from build123d import *

# Parameters (mm, degrees)
CYLINDER1189_R               = 1.5
CYLINDER1189_DEPTH           = 100
CYLINDER1190_R               = 1.5
CYLINDER1190_DEPTH           = 100
CYLINDER1187_R               = 1.5
CYLINDER1187_DEPTH           = 100
CYLINDER1188_R               = 1.5
CYLINDER1188_DEPTH           = 100
BOX491_W                     = 2
BOX491_H                     = 6
BOX491_DEPTH                 = 6
BOX492_W                     = 2
BOX492_H                     = 6
BOX492_DEPTH                 = 6
BOX493_W                     = 2
BOX493_H                     = 6
BOX493_DEPTH                 = 6
BOX490_W                     = 2
BOX490_H                     = 6
BOX490_DEPTH                 = 6
BOX460_W                     = 8
BOX460_H                     = 6
BOX460_DEPTH                 = 2
BOX460_PLACEMENT_ANGLE       = 45
BOX461_W                     = 8
BOX461_H                     = 6
BOX461_DEPTH                 = 2
BOX462_W                     = 8
BOX462_H                     = 6
BOX462_DEPTH                 = 2
BOX462_PLACEMENT_ANGLE       = 135
BOX463_W                     = 8
BOX463_H                     = 6
BOX463_DEPTH                 = 2
BOX464_W                     = 8
BOX464_H                     = 6
BOX464_DEPTH                 = 2
BOX464_PLACEMENT_ANGLE       = 225
BOX465_W                     = 8
BOX465_H                     = 6
BOX465_DEPTH                 = 2
BOX466_W                     = 8
BOX466_H                     = 6
BOX466_DEPTH                 = 2
BOX466_PLACEMENT_ANGLE       = 45
BOX459_W                     = 8
BOX459_H                     = 6
BOX459_DEPTH                 = 2
CYLINDER1161_R               = 1.5
CYLINDER1161_DEPTH           = 50
CYLINDER1161_PLACEMENT_ANGLE = 45
CYLINDER1162_R               = 1.5
CYLINDER1162_DEPTH           = 50
CYLINDER1163_R               = 1.5
CYLINDER1163_DEPTH           = 50
CYLINDER1163_PLACEMENT_ANGLE = 135
CYLINDER1164_R               = 1.5
CYLINDER1164_DEPTH           = 50
CYLINDER1165_R               = 1.5
CYLINDER1165_DEPTH           = 50
CYLINDER1165_PLACEMENT_ANGLE = 225
CYLINDER1166_R               = 1.5
CYLINDER1166_DEPTH           = 50
CYLINDER1167_R               = 1.5
CYLINDER1167_DEPTH           = 50
CYLINDER1167_PLACEMENT_ANGLE = 45
CYLINDER1160_R               = 1.5
CYLINDER1160_DEPTH           = 50
TUBE109_R                    = 50
TUBE109_R_2                  = 40
TUBE109_DEPTH                = 11
TUBE107_R                    = 54
TUBE107_R_2                  = 47
TUBE107_DEPTH                = 25


with BuildPart() as obj1:
    # Cylinder1189 → Cylinder1189 (new body)
    with BuildSketch(Plane(origin=(24, -51, 27), x_dir=(0, 0, -1), z_dir=(1, 0, 0))):
        Circle(CYLINDER1189_R)
    extrude(amount=CYLINDER1189_DEPTH)


with BuildPart() as obj2:
    # Cylinder1190 → Cylinder1190 (new body)
    with BuildSketch(Plane(origin=(34, 36, 42), x_dir=(0, 0, -1), z_dir=(1, 0, 0))):
        Circle(CYLINDER1190_R)
    extrude(amount=CYLINDER1190_DEPTH)


with BuildPart() as obj3:
    # Cylinder1187 → Cylinder1187 (new body)
    with BuildSketch(Plane(origin=(34, -36, 42), x_dir=(0, 0, -1), z_dir=(1, 0, 0))):
        Circle(CYLINDER1187_R)
    extrude(amount=CYLINDER1187_DEPTH)


with BuildPart() as compound890:
    # Cylinder1188 → Cylinder1188 (new body)
    with BuildSketch(Plane(origin=(24, 51, 27), x_dir=(0, 0, -1), z_dir=(1, 0, 0))):
        Circle(CYLINDER1188_R)
    extrude(amount=CYLINDER1188_DEPTH)

    # Compound890: union obj1, obj2, obj3
    add(obj1.part)
    add(obj2.part)
    add(obj3.part)


with BuildPart() as krychle491:
    # Box491 → Box491 (new body)
    with BuildSketch(Plane(origin=(32, -54, 24), x_dir=(1, 0, 0), z_dir=(0, 0, 1))):
        with Locations((1, 3)):
            Rectangle(BOX491_W, BOX491_H)
    extrude(amount=BOX491_DEPTH)


with BuildPart() as krychle492:
    # Box492 → Box492 (new body)
    with BuildSketch(Plane(origin=(38, 33, 39), x_dir=(1, 0, 0), z_dir=(0, 0, 1))):
        with Locations((1, 3)):
            Rectangle(BOX492_W, BOX492_H)
    extrude(amount=BOX492_DEPTH)


with BuildPart() as krychle493:
    # Box493 → Box493 (new body)
    with BuildSketch(Plane(origin=(38, -39, 39), x_dir=(1, 0, 0), z_dir=(0, 0, 1))):
        with Locations((1, 3)):
            Rectangle(BOX493_W, BOX493_H)
    extrude(amount=BOX493_DEPTH)


with BuildPart() as compound888:
    # Box490 → Box490 (new body)
    with BuildSketch(Plane(origin=(32, 48, 24), x_dir=(1, 0, 0), z_dir=(0, 0, 1))):
        with Locations((1, 3)):
            Rectangle(BOX490_W, BOX490_H)
    extrude(amount=BOX490_DEPTH)

    # Compound888: union Krychle491, Krychle492, Krychle493
    add(krychle491.part)
    add(krychle492.part)
    add(krychle493.part)


with BuildPart() as krychle460:
    # Box460 → Box460 (new body)
    with BuildSketch(Plane.XY):
        with Locations((4, 3)):
            Rectangle(BOX460_W, BOX460_H)
    extrude(amount=BOX460_DEPTH)


with BuildPart() as krychle460_1:
    # Box460 placement: moved
    add(krychle460.part.moved(Location((35.355339, 31.112698, 34))).rotate(Axis((35.355339, 31.112698, 34), (0, 0, 1)), BOX460_PLACEMENT_ANGLE))


with BuildPart() as krychle461:
    # Box461 → Box461 (new body)
    with BuildSketch(Plane(origin=(3, 47, 34), x_dir=(0, 1, 0), z_dir=(0, 0, 1))):
        with Locations((4, 3)):
            Rectangle(BOX461_W, BOX461_H)
    extrude(amount=BOX461_DEPTH)


with BuildPart() as krychle462:
    # Box462 → Box462 (new body)
    with BuildSketch(Plane.XY):
        with Locations((4, 3)):
            Rectangle(BOX462_W, BOX462_H)
    extrude(amount=BOX462_DEPTH)


with BuildPart() as krychle462_1:
    # Box462 placement: moved
    add(krychle462.part.moved(Location((-31.112698, 35.355339, 34))).rotate(Axis((-31.112698, 35.355339, 34), (0, 0, 1)), BOX462_PLACEMENT_ANGLE))


with BuildPart() as krychle463:
    # Box463 → Box463 (new body)
    with BuildSketch(Plane(origin=(-47, 3, 34), x_dir=(-1, 0, 0), z_dir=(0, 0, 1))):
        with Locations((4, 3)):
            Rectangle(BOX463_W, BOX463_H)
    extrude(amount=BOX463_DEPTH)


with BuildPart() as krychle464:
    # Box464 → Box464 (new body)
    with BuildSketch(Plane.XY):
        with Locations((4, 3)):
            Rectangle(BOX464_W, BOX464_H)
    extrude(amount=BOX464_DEPTH)


with BuildPart() as krychle464_1:
    # Box464 placement: moved
    add(krychle464.part.moved(Location((-35.355339, -31.112698, 34))).rotate(Axis((-35.355339, -31.112698, 34), (0, 0, 1)), BOX464_PLACEMENT_ANGLE))


with BuildPart() as krychle465:
    # Box465 → Box465 (new body)
    with BuildSketch(Plane(origin=(-3, -47, 34), x_dir=(0, -1, 0), z_dir=(0, 0, 1))):
        with Locations((4, 3)):
            Rectangle(BOX465_W, BOX465_H)
    extrude(amount=BOX465_DEPTH)


with BuildPart() as krychle466:
    # Box466 → Box466 (new body)
    with BuildSketch(Plane.XY):
        with Locations((4, 3)):
            Rectangle(BOX466_W, BOX466_H)
    extrude(amount=BOX466_DEPTH)


with BuildPart() as krychle466_1:
    # Box466 placement: moved
    add(krychle466.part.moved(Location((31.112698, -35.355339, 34))).rotate(Axis((31.112698, -35.355339, 34), (0, 0, -1)), BOX466_PLACEMENT_ANGLE))


with BuildPart() as compound881:
    # Box459 → Box459 (new body)
    with BuildSketch(Plane(origin=(47, -3, 34), x_dir=(1, 0, 0), z_dir=(0, 0, 1))):
        with Locations((4, 3)):
            Rectangle(BOX459_W, BOX459_H)
    extrude(amount=BOX459_DEPTH)

    # Compound881: union Krychle460, Krychle461, Krychle462, Krychle463, Krychle464, Krychle465, Krychle466
    add(krychle460_1.part)
    add(krychle461.part)
    add(krychle462_1.part)
    add(krychle463.part)
    add(krychle464_1.part)
    add(krychle465.part)
    add(krychle466_1.part)


with BuildPart() as compound881_1:
    # Compound881 placement: moved
    add(compound881.part.moved(Location((0, 0, 1))))


with BuildPart() as obj4:
    # Cylinder1161 → Cylinder1161 (new body)
    with BuildSketch(Plane.XY):
        Circle(CYLINDER1161_R)
    extrude(amount=CYLINDER1161_DEPTH)


with BuildPart() as obj4_1:
    # Cylinder1161 placement: moved
    add(obj4.part.moved(Location((36.769553, 36.769553, 0))).rotate(Axis((36.769553, 36.769553, 0), (0, 0, 1)), CYLINDER1161_PLACEMENT_ANGLE))


with BuildPart() as obj5:
    # Cylinder1162 → Cylinder1162 (new body)
    with BuildSketch(Plane(origin=(0, 52, 0), x_dir=(0, 1, 0), z_dir=(0, 0, 1))):
        Circle(CYLINDER1162_R)
    extrude(amount=CYLINDER1162_DEPTH)


with BuildPart() as obj6:
    # Cylinder1163 → Cylinder1163 (new body)
    with BuildSketch(Plane.XY):
        Circle(CYLINDER1163_R)
    extrude(amount=CYLINDER1163_DEPTH)


with BuildPart() as obj6_1:
    # Cylinder1163 placement: moved
    add(obj6.part.moved(Location((-36.769553, 36.769553, 0))).rotate(Axis((-36.769553, 36.769553, 0), (0, 0, 1)), CYLINDER1163_PLACEMENT_ANGLE))


with BuildPart() as obj7:
    # Cylinder1164 → Cylinder1164 (new body)
    with BuildSketch(Plane(origin=(-52, 0, 0), x_dir=(-1, 0, 0), z_dir=(0, 0, 1))):
        Circle(CYLINDER1164_R)
    extrude(amount=CYLINDER1164_DEPTH)


with BuildPart() as obj8:
    # Cylinder1165 → Cylinder1165 (new body)
    with BuildSketch(Plane.XY):
        Circle(CYLINDER1165_R)
    extrude(amount=CYLINDER1165_DEPTH)


with BuildPart() as obj8_1:
    # Cylinder1165 placement: moved
    add(obj8.part.moved(Location((-36.769553, -36.769553, 0))).rotate(Axis((-36.769553, -36.769553, 0), (0, 0, 1)), CYLINDER1165_PLACEMENT_ANGLE))


with BuildPart() as obj9:
    # Cylinder1166 → Cylinder1166 (new body)
    with BuildSketch(Plane(origin=(0, -52, 0), x_dir=(0, -1, 0), z_dir=(0, 0, 1))):
        Circle(CYLINDER1166_R)
    extrude(amount=CYLINDER1166_DEPTH)


with BuildPart() as obj10:
    # Cylinder1167 → Cylinder1167 (new body)
    with BuildSketch(Plane.XY):
        Circle(CYLINDER1167_R)
    extrude(amount=CYLINDER1167_DEPTH)


with BuildPart() as obj10_1:
    # Cylinder1167 placement: moved
    add(obj10.part.moved(Location((36.769553, -36.769553, 0))).rotate(Axis((36.769553, -36.769553, 0), (0, 0, -1)), CYLINDER1167_PLACEMENT_ANGLE))


with BuildPart() as compound879:
    # Cylinder1160 → Cylinder1160 (new body)
    with BuildSketch(Plane(origin=(52, 0, 0), x_dir=(1, 0, 0), z_dir=(0, 0, 1))):
        Circle(CYLINDER1160_R)
    extrude(amount=CYLINDER1160_DEPTH)

    # Compound879: union obj4, obj5, obj6, obj7, obj8, obj9, obj10
    add(obj4_1.part)
    add(obj5.part)
    add(obj6_1.part)
    add(obj7.part)
    add(obj8_1.part)
    add(obj9.part)
    add(obj10_1.part)


with BuildPart() as compound879_1:
    # Compound879 placement: moved
    add(compound879.part.moved(Location((0, 0, -7))))


with BuildPart() as tube109:
    # Tube109 → Tube109 (new body)
    with BuildSketch(Plane.XY.offset(20)):
        Circle(TUBE109_R)
        Circle(TUBE109_R_2, mode=Mode.SUBTRACT)
    extrude(amount=TUBE109_DEPTH)


with BuildPart() as cut444:
    # Tube107 → Tube107 (new body)
    with BuildSketch(Plane.XY.offset(20)):
        Circle(TUBE107_R)
        Circle(TUBE107_R_2, mode=Mode.SUBTRACT)
    extrude(amount=TUBE107_DEPTH)

    # Cut429: cut Tube109
    add(tube109.part, mode=Mode.SUBTRACT)

    # Cut431: cut Compound879
    add(compound879_1.part, mode=Mode.SUBTRACT)

    # Cut432: cut Compound881
    add(compound881_1.part, mode=Mode.SUBTRACT)

    # Cut442: cut Compound888
    add(compound888.part, mode=Mode.SUBTRACT)

    # Cut444: cut Compound890
    add(compound890.part, mode=Mode.SUBTRACT)


solid = cut444.part
Source: CAD feature listing. Evaluate the final solid. Frame: model axes, mm. A direction names the side the tool comes from. Coordinates: 2 decimals unless noted, no trailing zeros. Order: outer loops, then holes, each group sorted by start corner. A loop starts at its lowest first (then second) coordinate and runs counter-clockwise, first axis right, second up.
Item 1: Pull-direction query (X, two-part tool) for faces 1 (the face through (50.8, -0.9, 40)), 2 (the face through (-50, 0, 37)); classes: pulls with the +X half, pulls with the -X half, needs draft (parallel to the pull), parting line crosses it, or undercut.
Output values:
face 1: undercut
face 2: needs draft
Item 2: Cut plane D-D (y = -52). Return loops of the section in (x, z), plus the area to 3 significant figures.
Output values:
outline: (-14.56, 20) - (-1.5, 20) - (-1.5, 35) - (-3, 35) - (-3, 37) - (-1.5, 37) - (-1.5, 43) - (1.5, 43) - (1.5, 37) - (3, 37) - (3, 35) - (1.5, 35) - (1.5, 20) - (14.56, 20) - (14.56, 45) - (-14.56, 45) - close
area: 653 mm2
Item 3: Material intervals for line 1 (Y direction, x = 0, z = 41.5); line 2 (Z direction, x = 48.5, y = 1.5), sorted ascending.
Output values:
line 1: y = -54 to -53.5, -50.5 to -47, 47 to 50.5, 53.5 to 54
line 2: z = 31 to 35, 37 to 45
Item 4: Cut plane A-A (y = -20.5). Return loops of the section in (x, z).
Output values:
outline: (-49.96, 20) - (-45.6, 20) - (-45.6, 31) - (-42.29, 31) - (-42.29, 45) - (-49.96, 45) - close; (42.29, 31) - (45.6, 31) - (45.6, 20) - (49.96, 20) - (49.96, 45) - (42.29, 45) - close
Item 5: Cut plane B-B (x = -8.5). Return loops of the section in (y, z) (3 decimals), plus the area to 3 significant figures.
Output values:
outline: (-53.327, 20) - (-49.272, 20) - (-49.272, 31) - (-46.225, 31) - (-46.225, 45) - (-53.327, 45) - close; (46.225, 31) - (49.272, 31) - (49.272, 20) - (53.327, 20) - (53.327, 45) - (46.225, 45) - close
area: 288 mm2
Item 6: Set-up query: faces 3 (the face through (40, 34, 42)), 4 (the face through (35.53, -34.99, 43.11)), 5 (the face through (-50, 0, 35)), 6 (the face through (-50.8, 0.9, 40)), 7 (the face through (40, -34, 42)). Return all of +Z, -Z, +X, -X, +Y, -Y with unobstructed straight access to the full face (end or side cutting, diameter ignored); none if empty.
Output values:
face 3: +Z, +Y
face 4: +X
face 5: -X
face 6: -Z
face 7: +Z, -Y
Item 7: Cut plane C-C (z = 24.5). Count the separate pieces of the cut face and the enclosed holes in it, plus the area to 3 significant figures.
Output values:
separate pieces: 1
enclosed holes: 9
area: 1,250 mm2
Item 8: First-contact query: P1, Ø1, axis at x = -6.5, z = 37, coming from the +Y side; P2, Ø1.8, axis at x = 52, y = 0, coming from the -Z side; P3, Ø3, axis at x = 3, z = 27, coming from the +Y side; P4, Ø1.5, axis at x = -22.5, y = -38.5, coming from the +Z side. Flat tips, straight axial feed; report the tip coordinate or a pass-through.
Output values:
P1: stops at y = 53.67
P2: stops at z = 43
P3: stops at y = 53.98
P4: passes through
